CAD build for the part. Positions are in the model's coordinates, mm. Face numbers are marked on the shaded views. Give positions to 0.01 mm unless a question says otherwise; leave off trailing zeros. Write each loop counter-clockwise with the first axis right and the second up, starting at its lowest first coordinate (ties: lowest second). Pieces come first, ordered by that corner, then holes. Notation, with made-up numbers: (1.5, -9.75) - (39.5, -9.75) arc R17 cw to (39.5, -5.75) - close; hole circle Ø3 at (39.5, -30). An arc over 180 degrees is marked (long way). Put each result on its own line as item: value. Start each with the question number.
1. Cut at B-B on z = 29. List the corners of the cut face in (x, y).
2. Cut at C-C on x = -3.5. List the corners of the cut face in (y, z), and give its area (3 significant figures).
3. Mould opens along Y. For the marked faces 1, 2 and 3 say: +Y half, -Y half, draft (parallel to the pull), parting line (faces both ways), or undercut.
4. Wall check: line 1 (Z direction, x = 3.5, y = 0); line 2 (Y direction, x = -0.25, z = 40); line 3 (X direction, y = -1, z = 20). Give the ranges that are in metal, low to high.
5. Drop flat-ended pins along their axis: pin 1 (1 mm diameter, centred on y = -2, z = 30, fed in from -X); pin 2 (1 mm diameter, centred on x = 2.5, z = 5, fed in from +Y); pin 3 (1 mm diameter, centred on x = 1.5, z = 11, fed in from -Y). Give the stop position or say it passes through.
6. Cut at A-A on x = 0. List the corners of the cut face in (y, z).
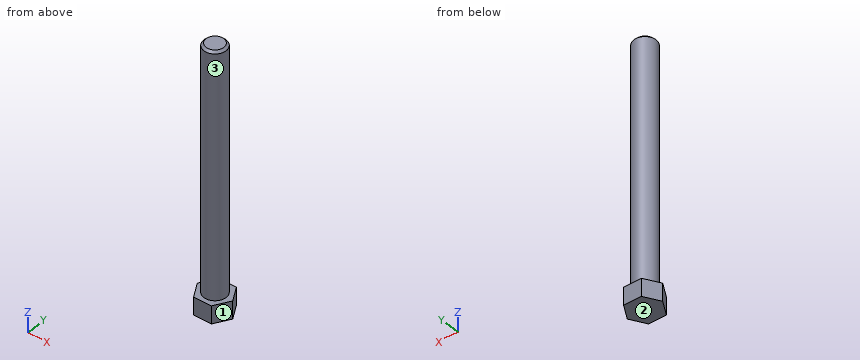
from build123d import *

# Parameters (mm, degrees)
SKETCH_1_R      = 2.5
EXTRUDE_1_DEPTH = 55
EXTRUDE_2_DEPTH = 4
CHAMFER_1_SIZE  = 0.5


with BuildPart() as part:
    # 草图1 → 拉伸1 (new body)
    with BuildSketch(Plane.XY):
        Circle(SKETCH_1_R)
    extrude(amount=EXTRUDE_1_DEPTH)

    # 草图2 → 拉伸2 (add)
    with BuildSketch(Plane.XY):
        Polygon((2, -3.464101615), (4, 0), (2, 3.464101615), (-2, 3.464101615), (-4, 0), (-2, -3.464101615), align=None)
    extrude(amount=-EXTRUDE_2_DEPTH)

    # 倒角1
    chamfer_1_edges = [part.edges().sort_by_distance(p)[0] for p in [
        (-2.5, 0, 55),
    ]]
    chamfer(chamfer_1_edges, length=CHAMFER_1_SIZE)


solid = part.part
Report:
1. outline: circle Ø5 at (0, 0)
2. outline: (-0.87, -4) - (0.87, -4) - (0.87, 0) - (-0.87, 0) - close
2. area: 6.93 mm²
3. face 1: -Y half
3. face 2: draft
3. face 3: parting line
4. line 1: z = -4 to 0
4. line 2: y = -2.49 to 2.49
4. line 3: x = -2.29 to 2.29
5. pin 1: stops at x = -2
5. pin 2: stops at y = 1.5
5. pin 3: stops at y = -2.29
6. outline: (-3.46, -4) - (3.46, -4) - (3.46, 0) - (2.5, 0) - (2.5, 54.5) - (2, 55) - (-2, 55) - (-2.5, 54.5) - (-2.5, 0) - (-3.46, 0) - close
